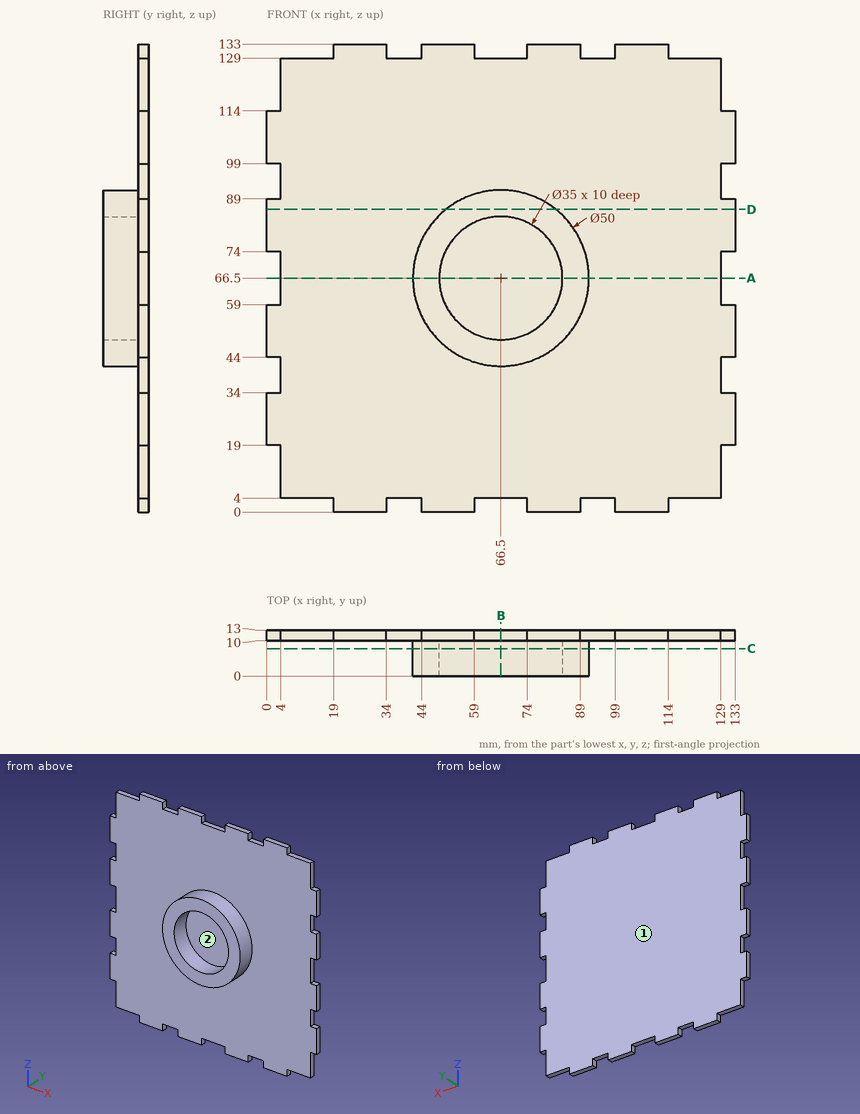
The figure shows three views and two pictorial views of one solid part (mm, origin at its lowest corner). Answer the questions. Coordinates: 2 decimals unless noted, no trailing zeros. Loops run counter-clockwise (first coordinate to the right, second up) from the corner with the lowest first, then second, coordinate; pieces in that order, holes last. Notation, with made-up numbers: (17, 84.25) -> (34, 84.25) arc R26 ccw to (34, 114.25) -> close; hole circle Ø4 at (44.5, 75.5). An arc over 180 degrees is marked (long way). Return JSON: item names as keys, results as strings. Group by question number.
(1) A cutting plane is placed at C-C on y = 7.75. Write down the section's boundary in (x, z), and give its area (3 significant figures).
(2) A cutting plane is placed at A-A on z = 66.5. Write down the section's boundary in (x, y), and give its area (3 significant figures).
(3) Given pin 1 Ø1.5 at (y, z) = (11.5, 132) entering from -X; pin 2 Ø3.5 at (x, y) = (131, 12) entering from +Z; pin 3 Ø2 at (x, y) = (59.5, 5.5) entering from +Z, each flat-ended and moving along its own axis, determine where each tip first touches the part or whether it passes through.
(4) Determine the mould class of the marked faces 1 and 2 for opening direction X: released by +X, released by -X, zero draft, split by the parting line, or undercut.
(5) A cutting plane is placed at B-B on x = 66.5. Write down the section's boundary in (y, z), and give its area (3 significant figures).
(6) A cutting plane is placed at D-D on z = 86. Write down the section's boundary in (x, y), and give its area (3 significant figures).
(7) Find the intervals of material crossed by probe 1 along Z at (x, y) = (66.5, 8.25); probe 2 along X at (y, z) = (12.5, 68.5); probe 3 along X at (y, z) = (2.75, 58.5), in increasing order. Write a range as from..to.
The answers:
{
 "1": {"outline": "circle Ø50 at (66.5, 66.5); hole circle Ø35 at (66.5, 66.5)", "area": "1,000 mm^2"},
 "2": {"outline": "(4, 10) -> (41.5, 10) -> (41.5, 0) -> (49, 0) -> (49, 10) -> (84, 10) -> (84, 0) -> (91.5, 0) -> (91.5, 10) -> (129, 10) -> (129, 13) -> (4, 13) -> close", "area": "525 mm^2"},
 "3": {"pin 1": "stops at x = 19", "pin 2": "stops at z = 114", "pin 3": "stops at z = 90.77"},
 "4": {"face 1": "zero draft", "face 2": "undercut"},
 "5": {"outline": "(0, 41.5) -> (10, 41.5) -> (10, 4) -> (13, 4) -> (13, 129) -> (10, 129) -> (10, 91.5) -> (0, 91.5) -> (0, 84) -> (10, 84) -> (10, 49) -> (0, 49) -> close", "area": "525 mm^2"},
 "6": {"outline": "(0, 10) -> (50.86, 10) -> (50.86, 0) -> (82.14, 0) -> (82.14, 10) -> (133, 10) -> (133, 13) -> (0, 13) -> close", "area": "712 mm^2"},
 "7": {"probe 1": "z = 41.5..49, 84..91.5", "probe 2": "x = 4..129", "probe 3": "x = 42.81..50.94, 82.06..90.19"}
}
